Could you check a few things on this model? Use its own coordinates, in mm. Give positions to 0.01 mm unless a question says otherwise; leave off trailing zeros. Order: outer loops, then holes, each group sorted by start corner. A loop starts at its lowest first (then second) coordinate and runs counter-clockwise, first axis right, second up. Notation, with made-up numbers: (55.5, -24) -> (76.5, -24) arc R14 ccw to (76.5, -1) -> close; hole circle Ø7 at (-25, -35.5). An arc over 180 degrees is marked (long way). Answer as CSV lines item,"result". Start each with the question number.
(1) Will these pins go through, and if not, where does the flat tip stop? pin 1 Ø4 at (x, z) = (-51, 3) entering from -Y; pin 2 Ø4 at (y, z) = (7, 3) entering from -X; pin 3 Ø2.5 at (y, z) = (5, 4) entering from +X; pin 4 Ø12 at (x, y) = (31.5, -8.5) entering from -Z.
(2) I want a section at D-D (x = 44). Please give me the cut outline in (y, z).
(3) I need wall thicknesses on L1, parallel to X at y = 2.5, z = 4; L2, parallel to Y at x = 22.5, z = 7.25; L3, parallel to X at y = -28, z = 7.25. Which ranges of each line are inside material? Lowest first, please.
(4) I want a section at A-A (y = -60). Please give me the cut outline in (x, z).
(5) I want a section at C-C (z = 6.75). Give the number of separate pieces and of enclosed holes in the cut face, plus the area to 3 significant figures.
(6) I want a section at B-B (y = -0.5). Please give me the cut outline in (x, z), plus the area to 3 significant figures.
```python
from build123d import *

# Parameters (mm, degrees)
SKETCH1_W           = 2
SKETCH1_H           = 20
SKETCH1_W_2         = 6
SKETCH1_H_2         = 10
BOSS_EXTRUDE1_DEPTH = 8
SKETCH3_W           = 8
SKETCH3_H           = 10
BOSS_EXTRUDE2_DEPTH = 8
SKETCH4_W           = 8
SKETCH4_H           = 10
BOSS_EXTRUDE3_DEPTH = 8


with BuildPart() as part:
    # Sketch1 → Boss-Extrude1 (new body)
    with BuildSketch(Plane.XY):
        with BuildLine():
            Line((-37.5, -87.5), (37.5, -87.5))
            ThreePointArc((37.5, -87.5), (44.571067812, -84.571067812), (47.5, -77.5))
            Line((47.5, -77.5), (47.5, 77.5))
            ThreePointArc((47.5, 77.5), (44.571067812, 84.571067812), (37.5, 87.5))
            Line((37.5, 87.5), (-37.5, 87.5))
            ThreePointArc((-37.5, 87.5), (-44.571067812, 84.571067812), (-47.5, 77.5))
            Line((-47.5, 77.5), (-47.5, -77.5))
            ThreePointArc((-47.5, -77.5), (-44.571067812, -84.571067812), (-37.5, -87.5))
        make_face()
        with Locations((-22.5, 0)):
            Rectangle(SKETCH1_W, SKETCH1_H, mode=Mode.SUBTRACT)
        with Locations((22.5, 0)):
            Rectangle(SKETCH1_W, SKETCH1_H, mode=Mode.SUBTRACT)
        with Locations((36.5, -62.5)):
            Rectangle(SKETCH1_W_2, SKETCH1_H_2, mode=Mode.SUBTRACT)
    extrude(amount=BOSS_EXTRUDE1_DEPTH)

    # Sketch3 → Boss-Extrude2 (add)
    with BuildSketch(Plane.ZY.offset(47.5)):
        with Locations((4, -62.5)):
            Rectangle(SKETCH3_W, SKETCH3_H)
        with Locations((4, -22.5)):
            Rectangle(SKETCH3_W, SKETCH3_H)
    extrude(amount=BOSS_EXTRUDE2_DEPTH)

    # Sketch4 → Boss-Extrude3 (add)
    with BuildSketch(Plane(origin=(47.5, 0, 0), x_dir=(0, 0, -1), z_dir=(1, 0, 0))):
        with Locations((-4, -62.5)):
            Rectangle(SKETCH4_W, SKETCH4_H)
        with Locations((-4, -32.5)):
            Rectangle(SKETCH4_W, SKETCH4_H)
    extrude(amount=BOSS_EXTRUDE3_DEPTH)


solid = part.part
```
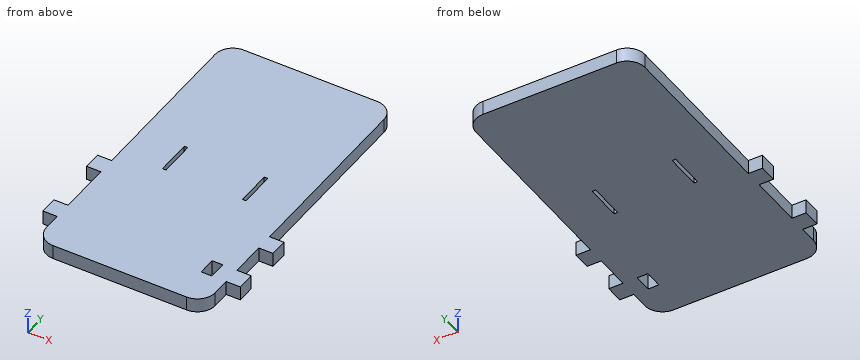
Final values:
1,pin 1,"y = -67.5"
1,pin 2,"x = -47.5"
1,pin 3,"x = 47.5"
1,pin 4,"z = 0"
2,outline,"(-85.1, 0) -> (85.1, 0) -> (85.1, 8) -> (-85.1, 8) -> close"
3,L1,"-47.5 to -23.5, -21.5 to 21.5, 23.5 to 47.5"
3,L2,"-87.5 to -10, 10 to 87.5"
3,L3,"-47.5 to 55.5"
4,outline,"(-55.5, 0) -> (33.5, 0) -> (33.5, 8) -> (-55.5, 8) -> close; (39.5, 0) -> (55.5, 0) -> (55.5, 8) -> (39.5, 8) -> close"
5,separate pieces,"1"
5,enclosed holes,"3"
5,area,"16,700 mm²"
6,outline,"(-47.5, 0) -> (-23.5, 0) -> (-23.5, 8) -> (-47.5, 8) -> close; (-21.5, 0) -> (21.5, 0) -> (21.5, 8) -> (-21.5, 8) -> close; (23.5, 0) -> (47.5, 0) -> (47.5, 8) -> (23.5, 8) -> close"
6,area,"728 mm²"
